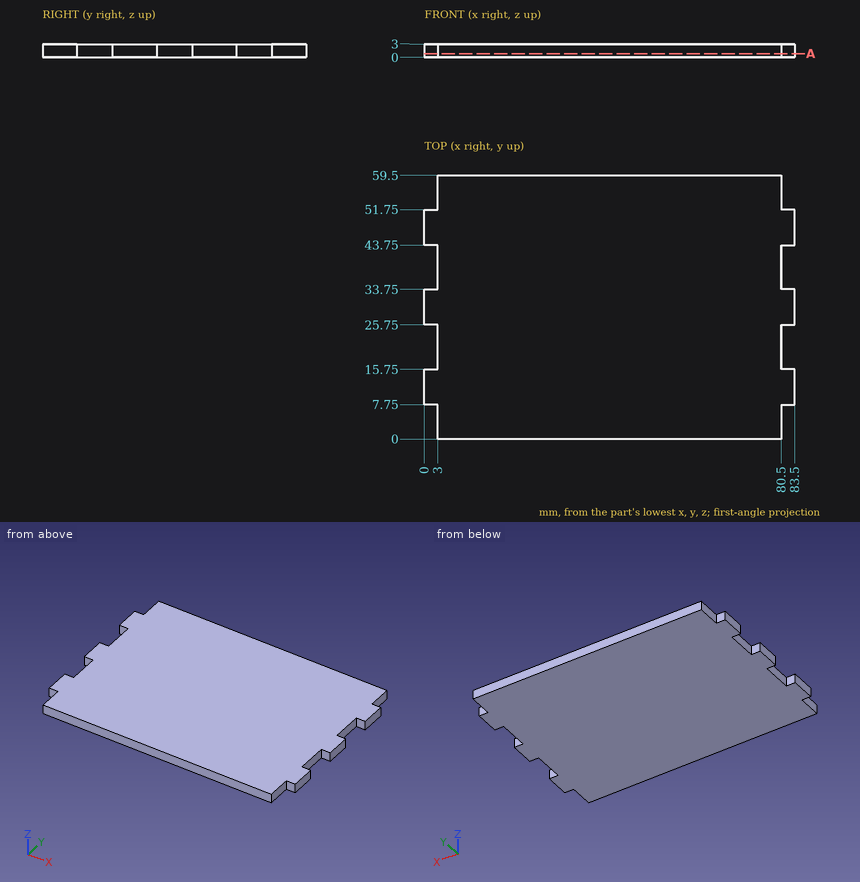
Study the drawing (mm; zero at the part's minimum x, y, z) and answer. Coordinates: 2 decimals unless noted, no trailing zeros. Loops run counter-clockwise (first coordinate to the right, second up) from the corner with the lowest first, then second, coordinate; pieces in that order, holes last. Notation, with made-up numbers: (58, 53.5) -> (102, 53.5) arc R15 cw to (102, 59.5) -> close; hole circle Ø10 at (20.5, -38.75). An arc over 180 degrees is marked (long way). Answer in a Markdown table with one row per item. Add a question column.
1. The part is cut by section A-A, the plane z = 0.85. Write down the section's boundary in (x, y), then the cut area to 3 significant figures.
2. Consider line 1 (X direction, y = 37, z = 1.55). Determine where the line is inside the solid, lowest interval first. Write a range as [from, to].
3. Flat-ended cylindrical pins translate along their axes: P1, Ø1.5, axis at x = 82, z = 1.5, coming from the +Y side; P2, Ø1.5, axis at x = 33.5, z = 1.5, coming from the -Y side; P3, Ø0.9, axis at x = 1, z = 1.5, coming from the -Y side; P4, Ø1.5, axis at y = 21.5, z = 2, coming from the -X side. Find the tip coordinate at first contact, or state that the pin passes through.
Answer below:
| question | item | result |
|---|---|---|
| 1 | outline | (0, 7.75) -> (3, 7.75) -> (3, 0) -> (80.5, 0) -> (80.5, 7.75) -> (83.5, 7.75) -> (83.5, 15.75) -> (80.5, 15.75) -> (80.5, 25.75) -> (83.5, 25.75) -> (83.5, 33.75) -> (80.5, 33.75) -> (80.5, 43.75) -> (83.5, 43.75) -> (83.5, 51.75) -> (80.5, 51.75) -> (80.5, 59.5) -> (3, 59.5) -> (3, 51.75) -> (0, 51.75) -> (0, 43.75) -> (3, 43.75) -> (3, 33.75) -> (0, 33.75) -> (0, 25.75) -> (3, 25.75) -> (3, 15.75) -> (0, 15.75) -> close |
| 1 | area | 4,760 mm2 |
| 2 | line 1 | [3, 80.5] |
| 3 | P1 | y = 51.75 |
| 3 | P2 | y = 0 |
| 3 | P3 | y = 7.75 |
| 3 | P4 | x = 3 |
